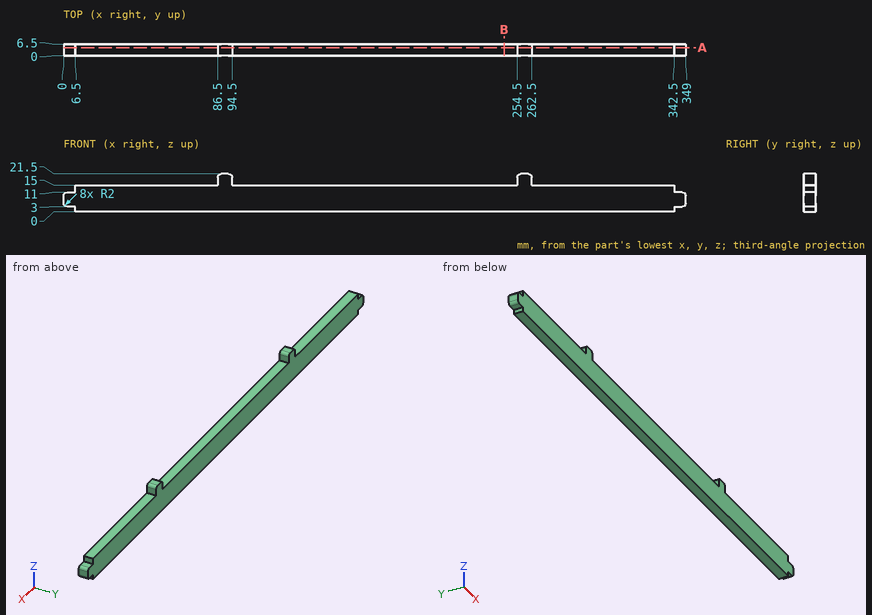
Job drawing, mm, ordinate dimensions from the low corner. One solid piece. Coordinates: 2 decimals unless noted, no trailing zeros. Order: outer loops, then holes, each group sorted by start corner. A loop starts at its lowest first (then second) coordinate and runs counter-clockwise, first axis right, second up. Notation, with made-up numbers: M 14.25,-15 L 42.25,-15 A16 ccw 42.25,4 Z; hole C 50.5,-7 d3. An arc over 180 degrees is marked long. Answer as CSV lines item,"result".
(1) Band-saw the part on A-A, the plane y = 4.5. List the corners of the cut face in (x, z).
Geometry says:
outline,"M 0,5 A2 ccw 2,3 L 6.5,3 L 6.5,0 L 342.5,0 L 342.5,3 L 347,3 A2 ccw 349,5 L 349,9 A2 ccw 347,11 L 342.5,11 L 342.5,15 L 262.5,15 L 262.5,19.5 A2 ccw 260.5,21.5 L 256.5,21.5 A2 ccw 254.5,19.5 L 254.5,15 L 94.5,15 L 94.5,19.5 A2 ccw 92.5,21.5 L 88.5,21.5 A2 ccw 86.5,19.5 L 86.5,15 L 6.5,15 L 6.5,11 L 2,11 A2 ccw 0,9 Z"
(2) Band-saw the part on B-B, the plane x = 247. List the corners of the cut face in (y, z).
Geometry says:
outline,"M 0,0 L 6.5,0 L 6.5,15 L 0,15 Z"
(3) Flat gauge pins, fed straight in: pin 1 (1.3 mm diameter, centred on x = 345, y = 2, fed in from -Z); pin 2 (2.5 mm diameter, centred on y = 3.5, z = 2, fed in from -X); pin 3 (3 mm diameter, centred on y = 2, z = 13, fed in from +X). Where does each tip first touch, or does it go through?
Geometry says:
pin 1,"stops at z = 3"
pin 2,"stops at x = 1.03"
pin 3,"stops at x = 342.5"
(4) Wall check: line 1 along X through (y, z) = (2.75, 16.25); line 2 along Z through (x, y) = (86, 4); line 3 along X through (y, z) = (5.75, 1.5). Give the ranges that are in metal, low to high.
Geometry says:
line 1,"x = 86.5 to 94.5, 254.5 to 262.5"
line 2,"z = 0 to 15"
line 3,"x = 6.5 to 342.5"
